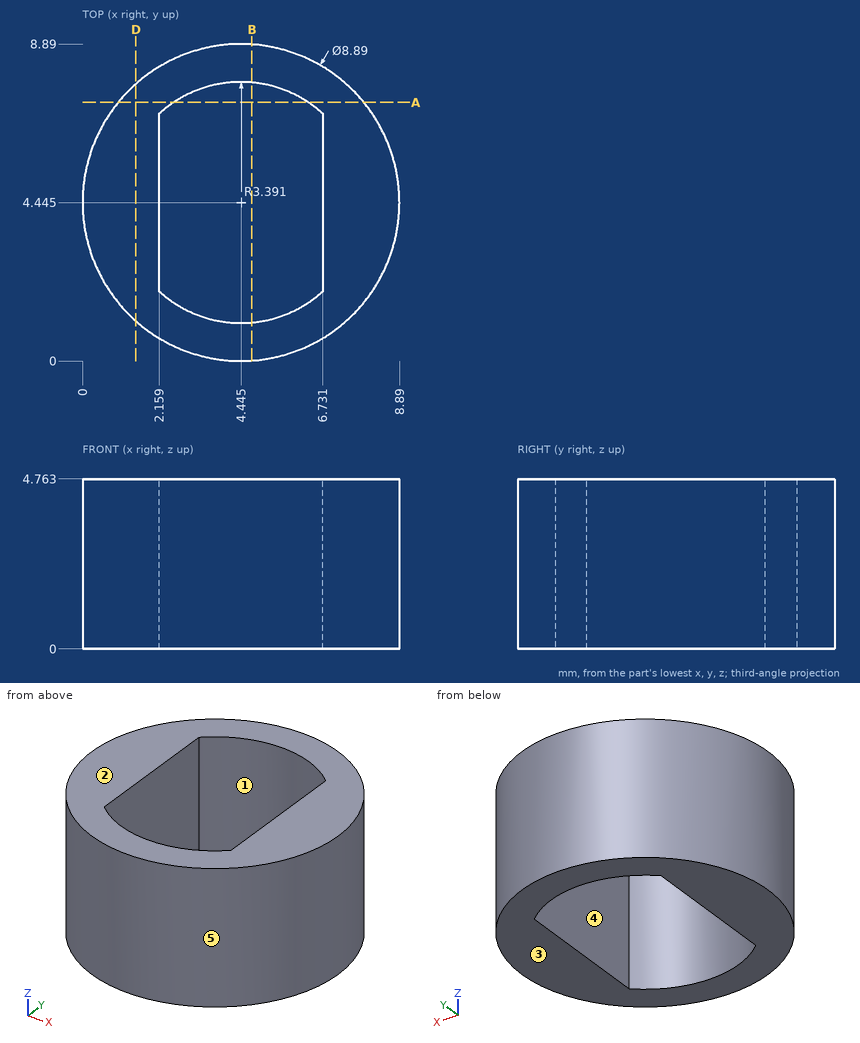
Here's the drawing with two shaded views (mm, measured from the low corner). I have some questions. A direction names the side the tool comes from. Coordinates: 2 decimals unless noted, no trailing zeros. Write each loop counter-clockwise with the first axis right and the second up, starting at its lowest first coordinate (ties: lowest second). Pieces come first, ordered by that corner, then holes. Notation, with made-up numbers: M -14,58.25 L 12,58.25 A12 ccw 12,64.25 Z; hole C 45.5,21 d4. An arc over 180 degrees is marked long. Answer as CSV lines item,"result". Start each with the question number.
1) Please list where these lines run through material, in increasing order: line 1 (Y direction, x = 3, z = 1.65); line 2 (X direction, y = 1.75, z = 2.55) (1 decimal); line 3 (X direction, y = 6.25, z = 2.75). Write a range as from..to.
2) I want a section at A-A, the plane y = 7.25. Please give me the cut outline in (x, z), and give its area (3 significant figures).
3) I want a section at B-B, the plane x = 4.75. Please give me the cut outline in (y, z).
4) We'd pull the mould along X, two halves only. Please class the marked faces 3, 4 and 5: +X half, -X half, draft (parallel to the pull), parting line (faces both ways), or undercut.
5) I want a section at D-D, the plane x = 1.5. Please give me the cut outline in (y, z) (1 decimal).
6) For the marked faces 1 and 2, which set-ups out of +Z, -Z, +X, -X, +Y, -Y let a thin tool reach every point of the face, with its end or its side?
7) For P1, Ø1.4, axis at y = 5.5, z = 1.5, coming from the +X side; P2, Ø1, axis at x = 2, z = 3, coming from the -Y side; P3, Ø3, axis at x = 4, y = 3.5, coming from the -Z side, each with a flat end and sliding along its axis, tell me the tip position at first contact or that it passes through.
Data:
1,line 1,"y = 0.24..1.38, 7.51..8.65"
1,line 2,"x = 0.9..2.4, 6.5..8"
1,line 3,"x = 0.38..2.16, 6.73..8.51"
2,outline,"M 1,0 L 2.54,0 L 2.54,4.76 L 1,4.76 Z; M 6.35,0 L 7.89,0 L 7.89,4.76 L 6.35,4.76 Z"
2,area,"14.7 mm^2"
3,outline,"M 0.01,0 L 1.07,0 L 1.07,4.76 L 0.01,4.76 Z; M 7.82,0 L 8.88,0 L 8.88,4.76 L 7.82,4.76 Z"
4,face 3,"draft"
4,face 4,"undercut"
4,face 5,"parting line"
5,outline,"M 1.1,0 L 7.8,0 L 7.8,4.8 L 1.1,4.8 Z"
6,face 1,"+Z, -Z"
6,face 2,"+Z, +X, -X, +Y, -Y"
7,P1,"stops at x = 8.88"
7,P2,"stops at y = 0.45"
7,P3,"passes through"
